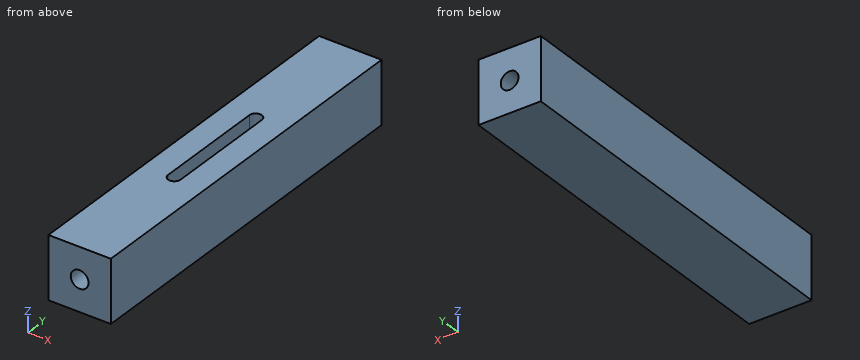
```python
from build123d import *

# Parameters (mm, degrees)
SKETCH2_W               = 24.9
SKETCH2_H               = 24.9
SKETCH2_R               = 3.55
BOSS_EXTRUDE1_DEPTH     = 150
CUT_EXTRUDE1_REACH      = 156.078
CUT_EXTRUDE1_END_RADIUS = 3.55


with BuildPart() as part:
    # Sketch2 → Boss-Extrude1 (new body)
    with BuildSketch(Plane(origin=(0, 0, 0), x_dir=(1, 0, 0), z_dir=(0, 1, 0))):
        with Locations((-12.45, 12.45)):
            Rectangle(SKETCH2_W, SKETCH2_H)
        with Locations(Location((-12.45, 12.45, 0), (0, 0, 270))):
            Circle(SKETCH2_R, mode=Mode.SUBTRACT)
    extrude(amount=BOSS_EXTRUDE1_DEPTH)

    # Cut-Extrude1: up to this cylinder (the profile starts outside it)
    cut_extrude1_end = Plane(origin=(-12.45, 75, -12.45), z_dir=(0, -1, 0)) * Cylinder(CUT_EXTRUDE1_END_RADIUS, 320.256, mode=Mode.PRIVATE)
    # Sketch3 → Cut-Extrude1 (cut, up to the surface)
    with BuildSketch(Plane.XY, mode=Mode.PRIVATE) as cut_extrude1_sk1:
        with BuildLine():
            Line((-14.95, 97.5), (-14.95, 52.5))
            ThreePointArc((-14.95, 52.5), (-12.45, 50), (-9.95, 52.5))
            Line((-9.95, 52.5), (-9.95, 97.5))
            ThreePointArc((-9.95, 97.5), (-12.45, 100), (-14.95, 97.5))
        make_face()
    cut_extrude1_tool1 = extrude(cut_extrude1_sk1.sketch, amount=-CUT_EXTRUDE1_REACH, mode=Mode.PRIVATE) - cut_extrude1_end
    add(cut_extrude1_tool1.solids().sort_by_distance((-12.45, 75, 0))[0], mode=Mode.SUBTRACT)


solid = part.part
```
Design review of the part built by this model. Coordinates are the model's own, in mm. Round coordinates to 2 decimals unless told otherwise and drop trailing zeros. Write each loop counter-clockwise with the first axis right and the second up, starting at its lowest first coordinate (ties: lowest second). Pieces come first, ordered by that corner, then holes. Notation, with made-up numbers: (-2, 26.5) -> (49, 26.5) arc R31 cw to (49, 59.5) -> close; hole circle Ø6 at (84.5, 31.25). An arc over 180 degrees is marked (long way). Answer in a Markdown table with one row per item.
Q1. To check wall thickness, follow L1, parallel to X at y = 60.5, z = -12.45; L2, parallel to Z at x = -12, y = 54; L3, parallel to Z at x = -10.5, y = 24.5. State the ranges of each line that lie inside material, in increasing order. Write a range as [from, to].
The answers:
| item | result |
|---|---|
| L1 | [-24.9, -16], [-8.9, 0] |
| L2 | [-24.9, -15.97] |
| L3 | [-24.9, -15.42], [-9.48, 0] |
Q2. Take a section at C-C, the plane z = -2.25. State the section outline as (x, y) points.
The answers:
| item | result |
|---|---|
| outline | (-24.9, 0) -> (0, 0) -> (0, 150) -> (-24.9, 150) -> close; hole (-14.95, 52.5) arc R2.5 ccw to (-9.95, 52.5) -> (-9.95, 97.5) arc R2.5 ccw to (-14.95, 97.5) -> close |
Q3. Take a section at A-A, the plane x = -12.45. State the section outline as (y, z) points, then the cut area to 4 significant figures.
The answers:
| item | result |
|---|---|
| outline | (0, -24.9) -> (150, -24.9) -> (150, -16) -> (0, -16) -> close; (0, -8.9) -> (50, -8.9) -> (50, 0) -> (0, 0) -> close; (100, -8.9) -> (150, -8.9) -> (150, 0) -> (100, 0) -> close |
| area | 2,225 mm² |
Q4. Clearance check with a flat-ended pin moving along its axis: pin 1 Ø1.5 at (x, y) = (-14, 27) entering from +Z. State where the tip first meets the part, or that it passes through.
The answers:
| item | result |
|---|---|
| pin 1 | z = 0 |
Q5. Take a section at B-B, the plane z = -12.45. State the section outline as (x, y) points.
The answers:
| item | result |
|---|---|
| outline | (-24.9, 0) -> (-16, 0) -> (-16, 150) -> (-24.9, 150) -> close; (-8.9, 0) -> (0, 0) -> (0, 150) -> (-8.9, 150) -> close |
Q6. Take a section at D-D, the plane y = 46. State the section outline as (x, z) points, then the cut area to 3 significant figures.
The answers:
| item | result |
|---|---|
| outline | (-24.9, -24.9) -> (0, -24.9) -> (0, 0) -> (-24.9, 0) -> close; hole circle Ø7.1 at (-12.45, -12.45) |
| area | 580 mm² |
